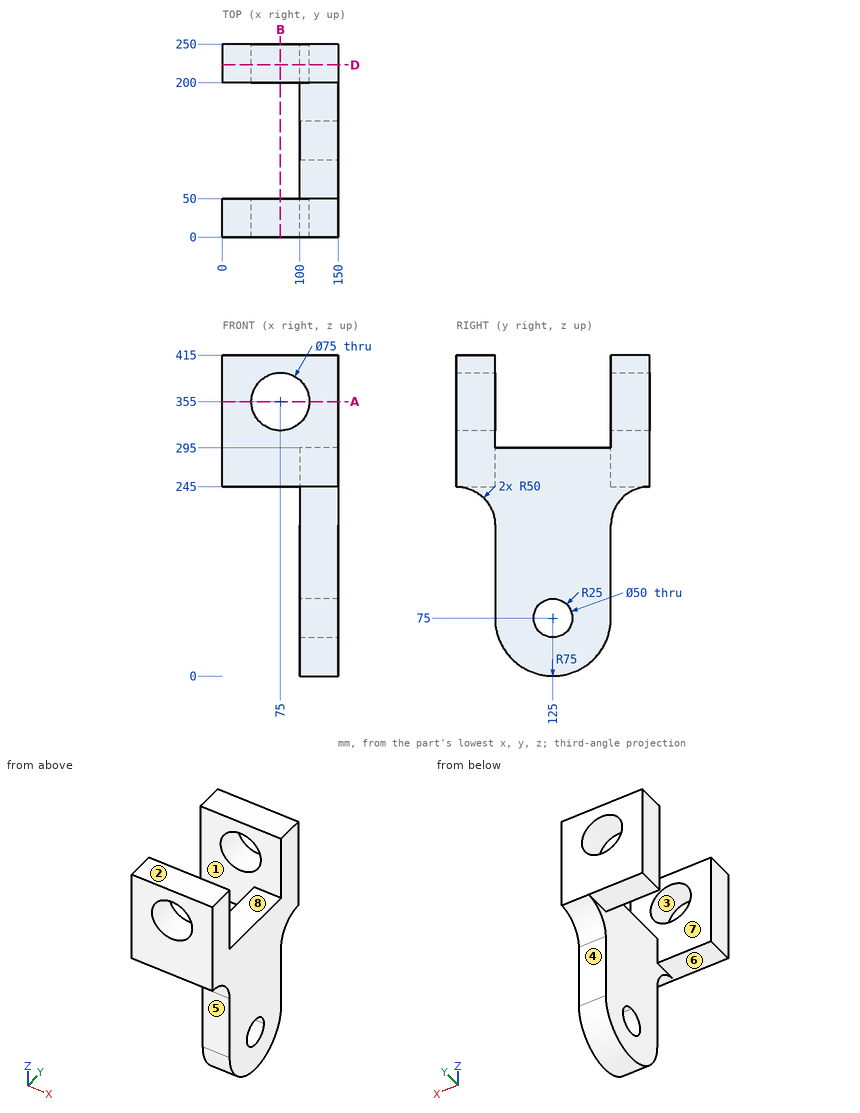
Answer from the drawing. Dimensions are ordinates in mm from the lowest x, y and z of the part. A direction names the side the tool comes from. Give positions to 0.01 mm unless a question says otherwise; leave off trailing zeros. Order: outer loops, then holes, each group sorted by start corner. A loop starts at its lowest first (then second) coordinate and runs counter-clockwise, first axis right, second up.
(1) Straight lines are drawn through the part: L1, parallel to Z at x = 75, y = 32; L2, parallel to Z at x = 120, y = 125; L3, parallel to Y at x = 91, z = 316.5. For each, find the intervals that lie inside material, in ascending order.
(2) Find section B-B (x = 75). Give the vertices of the cut face in (y, z).
(3) Given pin 1 (25 mm diameter, centred on x = 131.5, z = 130, fed in from -Y); pin 2 (10 mm diameter, centred on y = 127.5, z = 153, fed in from -X), each flat-ended and moving along its own axis, determine where each tip first touches the part or whether it passes through.
(4) Find section D-D (y = 223). Give the vertices of the cut face in (x, z).
(5) For a pull along Z with two mould halves and no side action, classify the marked faces 1, 2 and 3 as released by +Z, released by -Z, zero draft, split by the parting line, or undercut.
(6) For the marked faces 4, 5, 6, 7 and 8, determine the directions among +Z, -Z, +X, -X, +Y, -Y from which every point of the face is accessible in a straight line to the end or side of a thin tool.
(7) Find section A-A (z = 355). Give the vertices of the cut face in (x, y), plus the area to 3 significant figures.
Result sheet:
1. L1: z = 245 to 317.5, 392.5 to 415
1. L2: z = 0 to 50, 100 to 295
1. L3: y = 0 to 50, 200 to 250
2. outline: (0, 245) - (50, 245) - (50, 317.5) - (0, 317.5) - close; (0, 392.5) - (50, 392.5) - (50, 415) - (0, 415) - close; (200, 245) - (250, 245) - (250, 317.5) - (200, 317.5) - close; (200, 392.5) - (250, 392.5) - (250, 415) - (200, 415) - close
3. pin 1: stops at y = 50
3. pin 2: stops at x = 100
4. outline: (0, 245) - (100, 245) - (100, 237.08) - (150, 237.08) - (150, 415) - (0, 415) - close; hole circle Ø75 at (75, 355)
5. face 1: zero draft
5. face 2: released by +Z
5. face 3: undercut
6. face 4: -Z, +X, -X, +Y
6. face 5: -Z, +X, -X, -Y
6. face 6: -Z, -X, +Y, -Y
6. face 7: +Z, -X
6. face 8: +Z, +X, -X
7. outline: (0, 0) - (37.5, 0) - (37.5, 50) - (0, 50) - close; (0, 200) - (37.5, 200) - (37.5, 250) - (0, 250) - close; (112.5, 0) - (150, 0) - (150, 50) - (112.5, 50) - close; (112.5, 200) - (150, 200) - (150, 250) - (112.5, 250) - close
7. area: 7,500 mm2
